from build123d import *

# Parameters (mm, degrees)
SKETCH1_W               = 150
SKETCH1_H               = 100
BOSS_EXTRUDE1_DEPTH     = 3
SKETCH2_W               = 10
SKETCH2_H               = 3
CUT_EXTRUDE2_DEPTH      = 91.188691087
LPATTERN1_COUNT         = 8
LPATTERN1_PITCH         = 20
MIRROR1_COPY_1_SKETCH_W = 10
MIRROR1_COPY_1_SKETCH_H = 3
MIRROR1_COPY_1_DEPTH    = 91.188691087
MIRROR1_COPY_2_SKETCH_W = 10
MIRROR1_COPY_2_SKETCH_H = 3
MIRROR1_COPY_2_DEPTH    = 91.188691087
MIRROR1_COPY_3_SKETCH_W = 10
MIRROR1_COPY_3_SKETCH_H = 3
MIRROR1_COPY_3_DEPTH    = 91.188691087
MIRROR1_COPY_4_SKETCH_W = 10
MIRROR1_COPY_4_SKETCH_H = 3
MIRROR1_COPY_4_DEPTH    = 91.188691087
MIRROR1_COPY_5_SKETCH_W = 10
MIRROR1_COPY_5_SKETCH_H = 3
MIRROR1_COPY_5_DEPTH    = 91.188691087
MIRROR1_COPY_6_SKETCH_W = 10
MIRROR1_COPY_6_SKETCH_H = 3
MIRROR1_COPY_6_DEPTH    = 91.188691087
MIRROR1_COPY_7_SKETCH_W = 10
MIRROR1_COPY_7_SKETCH_H = 3
MIRROR1_COPY_7_DEPTH    = 91.188691087
SKETCH3_W               = 3
SKETCH3_H               = 10
CUT_EXTRUDE3_DEPTH      = 91.188691087
LPATTERN2_COUNT         = 5
LPATTERN2_PITCH         = 20
MIRROR2_COPY_1_SKETCH_W = 3
MIRROR2_COPY_1_SKETCH_H = 10
MIRROR2_COPY_1_DEPTH    = 91.188691087
MIRROR2_COPY_2_SKETCH_W = 3
MIRROR2_COPY_2_SKETCH_H = 10
MIRROR2_COPY_2_DEPTH    = 91.188691087
MIRROR2_COPY_3_SKETCH_W = 3
MIRROR2_COPY_3_SKETCH_H = 10
MIRROR2_COPY_3_DEPTH    = 91.188691087
MIRROR2_COPY_4_SKETCH_W = 3
MIRROR2_COPY_4_SKETCH_H = 10
MIRROR2_COPY_4_DEPTH    = 91.188691087
SKETCH4_W               = 40
SKETCH4_H               = 20
CUT_EXTRUDE4_DEPTH      = 91.188691087
FILLET1_R               = 10
SKETCH5_W               = 3
SKETCH5_H               = 3
BOSS_EXTRUDE2_DEPTH     = 3
SKETCH6_R               = 1.5
SKETCH6_R_2             = 1.25
CUT_EXTRUDE5_DEPTH      = 91.188691087


with BuildPart() as part:
    # Sketch1 → Boss-Extrude1 (new body)
    with BuildSketch(Plane(origin=(0, 0, 0), x_dir=(1, 0, 0), z_dir=(0, 1, 0))):
        Rectangle(SKETCH1_W, SKETCH1_H)
    extrude(amount=BOSS_EXTRUDE1_DEPTH)

    # Sketch2 → Cut-Extrude2 (cut, through all)
    with BuildSketch(Plane(origin=(0, 3, 0), x_dir=(1, 0, 0), z_dir=(0, 1, 0))):
        with Locations((-70, -48.5)):
            Rectangle(SKETCH2_W, SKETCH2_H)
    cut_extrude2 = extrude(amount=-CUT_EXTRUDE2_DEPTH, mode=Mode.SUBTRACT)

    # LPattern1: Cut-Extrude2 ×8
    with Locations(*[(i * LPATTERN1_PITCH, 0, 0) for i in range(1, LPATTERN1_COUNT)]):
        add(cut_extrude2, mode=Mode.SUBTRACT)

    # Mirror1: Cut-Extrude2 across plane
    add(cut_extrude2.mirror(Plane.XY), mode=Mode.SUBTRACT)

    # Mirror1 copy 1 sketch → Mirror1 copy 1 (cut, through all)
    with BuildSketch(Plane(origin=(20, 3, 0), x_dir=(1, 0, 0), z_dir=(0, 1, 0))):
        with Locations((-70, 48.5)):
            Rectangle(MIRROR1_COPY_1_SKETCH_W, MIRROR1_COPY_1_SKETCH_H)
    extrude(amount=-MIRROR1_COPY_1_DEPTH, mode=Mode.SUBTRACT)

    # Mirror1 copy 2 sketch → Mirror1 copy 2 (cut, through all)
    with BuildSketch(Plane(origin=(40, 3, 0), x_dir=(1, 0, 0), z_dir=(0, 1, 0))):
        with Locations((-70, 48.5)):
            Rectangle(MIRROR1_COPY_2_SKETCH_W, MIRROR1_COPY_2_SKETCH_H)
    extrude(amount=-MIRROR1_COPY_2_DEPTH, mode=Mode.SUBTRACT)

    # Mirror1 copy 3 sketch → Mirror1 copy 3 (cut, through all)
    with BuildSketch(Plane(origin=(60, 3, 0), x_dir=(1, 0, 0), z_dir=(0, 1, 0))):
        with Locations((-70, 48.5)):
            Rectangle(MIRROR1_COPY_3_SKETCH_W, MIRROR1_COPY_3_SKETCH_H)
    extrude(amount=-MIRROR1_COPY_3_DEPTH, mode=Mode.SUBTRACT)

    # Mirror1 copy 4 sketch → Mirror1 copy 4 (cut, through all)
    with BuildSketch(Plane(origin=(80, 3, 0), x_dir=(1, 0, 0), z_dir=(0, 1, 0))):
        with Locations((-70, 48.5)):
            Rectangle(MIRROR1_COPY_4_SKETCH_W, MIRROR1_COPY_4_SKETCH_H)
    extrude(amount=-MIRROR1_COPY_4_DEPTH, mode=Mode.SUBTRACT)

    # Mirror1 copy 5 sketch → Mirror1 copy 5 (cut, through all)
    with BuildSketch(Plane(origin=(100, 3, 0), x_dir=(1, 0, 0), z_dir=(0, 1, 0))):
        with Locations((-70, 48.5)):
            Rectangle(MIRROR1_COPY_5_SKETCH_W, MIRROR1_COPY_5_SKETCH_H)
    extrude(amount=-MIRROR1_COPY_5_DEPTH, mode=Mode.SUBTRACT)

    # Mirror1 copy 6 sketch → Mirror1 copy 6 (cut, through all)
    with BuildSketch(Plane(origin=(120, 3, 0), x_dir=(1, 0, 0), z_dir=(0, 1, 0))):
        with Locations((-70, 48.5)):
            Rectangle(MIRROR1_COPY_6_SKETCH_W, MIRROR1_COPY_6_SKETCH_H)
    extrude(amount=-MIRROR1_COPY_6_DEPTH, mode=Mode.SUBTRACT)

    # Mirror1 copy 7 sketch → Mirror1 copy 7 (cut, through all)
    with BuildSketch(Plane(origin=(140, 3, 0), x_dir=(1, 0, 0), z_dir=(0, 1, 0))):
        with Locations((-70, 48.5)):
            Rectangle(MIRROR1_COPY_7_SKETCH_W, MIRROR1_COPY_7_SKETCH_H)
    extrude(amount=-MIRROR1_COPY_7_DEPTH, mode=Mode.SUBTRACT)

    # Sketch3 → Cut-Extrude3 (cut, through all)
    with BuildSketch(Plane(origin=(0, 3, 0), x_dir=(1, 0, 0), z_dir=(0, 1, 0))):
        with Locations((-73.5, -35)):
            Rectangle(SKETCH3_W, SKETCH3_H)
    cut_extrude3 = extrude(amount=-CUT_EXTRUDE3_DEPTH, mode=Mode.SUBTRACT)

    # LPattern2: Cut-Extrude3 ×5
    with Locations(*[(0, 0, -i * LPATTERN2_PITCH) for i in range(1, LPATTERN2_COUNT)]):
        add(cut_extrude3, mode=Mode.SUBTRACT)

    # Mirror2: Cut-Extrude3 across plane
    add(cut_extrude3.mirror(Plane(origin=(0, 0, 0), x_dir=(0, 0, 1), z_dir=(1, 0, 0))), mode=Mode.SUBTRACT)

    # Mirror2 copy 1 sketch → Mirror2 copy 1 (cut, through all)
    with BuildSketch(Plane(origin=(0, 3, -20), x_dir=(-1, 0, 0), z_dir=(0, 1, 0))):
        with Locations((-73.5, 35)):
            Rectangle(MIRROR2_COPY_1_SKETCH_W, MIRROR2_COPY_1_SKETCH_H)
    extrude(amount=-MIRROR2_COPY_1_DEPTH, mode=Mode.SUBTRACT)

    # Mirror2 copy 2 sketch → Mirror2 copy 2 (cut, through all)
    with BuildSketch(Plane(origin=(0, 3, -40), x_dir=(-1, 0, 0), z_dir=(0, 1, 0))):
        with Locations((-73.5, 35)):
            Rectangle(MIRROR2_COPY_2_SKETCH_W, MIRROR2_COPY_2_SKETCH_H)
    extrude(amount=-MIRROR2_COPY_2_DEPTH, mode=Mode.SUBTRACT)

    # Mirror2 copy 3 sketch → Mirror2 copy 3 (cut, through all)
    with BuildSketch(Plane(origin=(0, 3, -60), x_dir=(-1, 0, 0), z_dir=(0, 1, 0))):
        with Locations((-73.5, 35)):
            Rectangle(MIRROR2_COPY_3_SKETCH_W, MIRROR2_COPY_3_SKETCH_H)
    extrude(amount=-MIRROR2_COPY_3_DEPTH, mode=Mode.SUBTRACT)

    # Mirror2 copy 4 sketch → Mirror2 copy 4 (cut, through all)
    with BuildSketch(Plane(origin=(0, 3, -80), x_dir=(-1, 0, 0), z_dir=(0, 1, 0))):
        with Locations((-73.5, 35)):
            Rectangle(MIRROR2_COPY_4_SKETCH_W, MIRROR2_COPY_4_SKETCH_H)
    extrude(amount=-MIRROR2_COPY_4_DEPTH, mode=Mode.SUBTRACT)

    # Sketch4 → Cut-Extrude4 (cut, through all)
    with BuildSketch(Plane(origin=(0, 3, 0), x_dir=(1, 0, 0), z_dir=(0, 1, 0))):
        with Locations((-10, 27.5)):
            Rectangle(SKETCH4_W, SKETCH4_H)
    extrude(amount=-CUT_EXTRUDE4_DEPTH, mode=Mode.SUBTRACT)

    # Fillet1
    fillet1_edges = [part.edges().sort_by_distance(p)[0] for p in [
        (10, 1.5, -17.5),
        (10, 1.5, -37.5),
        (-30, 1.5, -37.5),
        (-30, 1.5, -17.5),
    ]]
    fillet(fillet1_edges, radius=FILLET1_R - 0.0001)  # a hair under: the kernel refuses the full size

    # Sketch5 → Boss-Extrude2 (add)
    with BuildSketch(Plane.XY.offset(47)):
        with Locations((73.5, 1.5)):
            Rectangle(SKETCH5_W, SKETCH5_H)
    boss_extrude2 = extrude(amount=BOSS_EXTRUDE2_DEPTH)

    # Mirror3: Boss-Extrude2 across plane
    add(boss_extrude2.mirror(Plane(origin=(0, 0, 0), x_dir=(0, 0, 1), z_dir=(1, 0, 0))))

    # Sketch6 → Cut-Extrude5 (cut, through all)
    with BuildSketch(Plane(origin=(0, 3, 0), x_dir=(1, 0, 0), z_dir=(0, 1, 0))):
        with Locations(Location((-13.16772538, -36.12518928, 0), (0, 0, 270))):
            Circle(SKETCH6_R)
        with Locations(Location((-13.16772538, 5.78481072, 0), (0, 0, 270))):
            Circle(SKETCH6_R)
        with Locations(Location((52.87227462, 8.95981072, 0), (0, 0, 270))):
            Circle(SKETCH6_R)
        with Locations(Location((52.87227462, -39.30018928, 0), (0, 0, 270))):
            Circle(SKETCH6_R)
        with Locations(Location((-39.54, -39.96, 0), (0, 0, 270))):
            Circle(SKETCH6_R_2)
        with Locations(Location((-62.4, -39.96, 0), (0, 0, 270))):
            Circle(SKETCH6_R_2)
        with Locations(Location((-62.4, 8.3, 0), (0, 0, 270))):
            Circle(SKETCH6_R_2)
    extrude(amount=-CUT_EXTRUDE5_DEPTH, mode=Mode.SUBTRACT)


solid = part.part
Here's how the part is built. I have some questions about the finished solid (model axes, mm). A direction names the side the tool comes from. Coordinates: 2 decimals unless noted, no trailing zeros. Loops run counter-clockwise (first coordinate to the right, second up) from the corner with the lowest first, then second, coordinate; pieces in that order, holes last. Notation, with made-up numbers: (-24.75, -7) -> (-11.75, -7) arc R14 ccw to (-11.75, 6) -> close; hole circle Ø4 at (-2.5, 6.25). An arc over 180 degrees is marked (long way). Use one line per item in the form item = value. Start each with the question number.
(1) If we section it at B-B (y = 2.5): Give the number of separate pieces and of enclosed holes in the cut face, then the cut area to 3 significant figures.
(2) Please list where these lines run through material, in increasing order: line 1 along X through (y, z) = (1.25, -8.3); line 2 along X through (y, z) = (1.6, 41); line 3 along X through (y, z) = (2.35, 39.96).
(3) On a 3-axis mill with a long thin cutter (end or side, diameter ignored), from which of +Z, -Z, +X, -X, +Y, -Y can I reach the whole of each face in a straight line? I mean faces 1 (the face through (-50, 2, -47)), 2 (the face through (-30, 2, 47)), 3 (the face through (72, 2, 15)), 4 (the face through (-74, 2, -20)). Say none if no direction works.
(4) Will these pins go through, and if not, where does the flat tip stop? pin 1 (4 mm diameter, centred on x = 52.87, z = 39.3, fed in from -Y); pin 2 (0.9 mm diameter, centred on y = 2, z = 36.5, fed in from +X); pin 3 (2.5 mm diameter, centred on x = 52.87, z = -8.96, fed in from +Y); pin 4 (0.9 mm diameter, centred on x = -11.5, y = 2, fed in from +Z).
(5) We'd pull the mould along X, two halves only. Please class faces 5 (the face through (75, 1, 25)), 6 (the face through (55, 2, -48)), 7 (the face through (73, 2, 50)): pulls with the +X half, pulls with the -X half, needs draft (parallel to the pull), parting line crosses it, or undercut.
(6) If we section it at A-A (x = -22): Please give me the cut outline in (y, z).
(7) If we section it at C-C (z = 18): Please give me the cut outline in (x, y).
Verdict:
q1.separate_pieces = 1
q1.enclosed_holes = 8
q1.area = 13,500 mm²
q2.line_1 = -72 to -63.65, -61.15 to 51.53, 54.22 to 72
q2.line_2 = -75 to -63.09, -61.71 to -40.23, -38.85 to 75
q2.line_3 = -72 to -63.65, -61.15 to -40.79, -38.29 to 51.53, 54.22 to 72
q3.face_1 = -Z, +Y, -Y
q3.face_2 = +Z, +Y, -Y
q3.face_3 = +X, +Y, -Y
q3.face_4 = -X, +Y, -Y
q4.pin_1 = 0
q4.pin_2 = 72
q4.pin_3 = through
q4.pin_4 = 47
q5.face_5 = pulls with the +X half
q5.face_6 = undercut
q5.face_7 = needs draft
q6.outline = (0, -50) -> (3, -50) -> (3, -37.3) -> (0, -37.3) -> close; (0, -17.7) -> (3, -17.7) -> (3, 50) -> (0, 50) -> close
q7.outline = (-72, 0) -> (72, 0) -> (72, 3) -> (-72, 3) -> close
